```python
from build123d import *

# Parameters (mm, degrees)
BOSS_EXTRUDE3_DEPTH = 50
SKETCH7_R           = 30
BOSS_EXTRUDE4_DEPTH = 100
BOSS_EXTRUDE7_DEPTH = 500
SKETCH9_R           = 25
CUT_EXTRUDE1_DEPTH  = 500
CUT_EXTRUDE2_START  = -500
CUT_EXTRUDE2_DEPTH  = 500
FILLET1_R           = 10
SKETCH12_W          = 100
SKETCH12_H          = 20
BOSS_EXTRUDE8_DEPTH = 40
CUT_EXTRUDE3_DEPTH  = 40
SKETCH14_R          = 10
CUT_EXTRUDE4_DEPTH  = 40


with BuildPart() as part:
    # Sketch3 → Boss-Extrude3 (new body)
    with BuildSketch(Plane(origin=(0, 0, 0), x_dir=(0, 0, -1), z_dir=(1, 0, 0))):
        with BuildLine():
            Line((0, 30), (100, 30))
            ThreePointArc((100, 30), (130, 0), (100, -30))
            Line((100, -30), (0, -30))
            ThreePointArc((0, -30), (-30, 0), (0, 30))
        make_face()
    extrude(amount=BOSS_EXTRUDE3_DEPTH)

    # Sketch7 → Boss-Extrude4 (add)
    with BuildSketch(Plane(origin=(50, 0, 0), x_dir=(0, 0, -1), z_dir=(1, 0, 0))):
        with Locations(Location((100, 0, 0), (0, 0, 90))):
            Circle(SKETCH7_R)
    extrude(amount=BOSS_EXTRUDE4_DEPTH)

    # Sketch8 → Boss-Extrude7 (add)
    with BuildSketch(Plane(origin=(50, 0, 0), x_dir=(0, 0, -1), z_dir=(1, 0, 0))):
        with BuildLine():
            Line((0, 30), (20, 30))
            ThreePointArc((20, 30), (50, 0), (20, -30))
            Line((20, -30), (0, -30))
            ThreePointArc((0, -30), (-30, 0), (0, 30))
        make_face()
    extrude(amount=BOSS_EXTRUDE7_DEPTH)

    # Sketch9 → Cut-Extrude1 (cut)
    with BuildSketch(Plane(origin=(550, 0, 0), x_dir=(0, 0, -1), z_dir=(1, 0, 0))):
        with Locations((20, 0)):
            Circle(SKETCH9_R)
    extrude(amount=-CUT_EXTRUDE1_DEPTH, mode=Mode.SUBTRACT)

    # Sketch10 → Cut-Extrude2 (cut)
    with BuildSketch(Plane(origin=(550, 0, 0), x_dir=(0, 0, -1), z_dir=(1, 0, 0)).offset(CUT_EXTRUDE2_START)):
        with BuildLine():
            ThreePointArc((0, 30), (-15.932656638, 25.419489618), (-27, 13.076696831))
            Line((-27, 13.076696831), (12.529758535, 30))
            Line((12.529758535, 30), (0, 30))
        make_face()
        with BuildLine():
            Line((12.529758535, -30), (-27, -13.076696831))
            ThreePointArc((-27, -13.076696831), (-15.932656638, -25.419489618), (0, -30))
            Line((0, -30), (12.529758535, -30))
        make_face()
        with BuildLine():
            Line((-27, 0), (-27, 13.076696831))
            ThreePointArc((-27, 13.076696831), (-29.240383034, 6.708203932), (-30, 0))
            Line((-30, 0), (-27, 0))
        make_face()
        with BuildLine():
            Line((-27, -13.076696831), (-27, 0))
            Line((-27, 0), (-30, 0))
            ThreePointArc((-30, 0), (-29.240383034, -6.708203932), (-27, -13.076696831))
        make_face()
        with BuildLine():
            Line((-27, 0), (-27, 13.076696831))
            ThreePointArc((-27, 13.076696831), (-29.240383034, 6.708203932), (-30, 0))
            Line((-30, 0), (-27, 0))
        make_face()
        with BuildLine():
            Line((-27, -13.076696831), (-27, 0))
            Line((-27, 0), (-30, 0))
            ThreePointArc((-30, 0), (-29.240383034, -6.708203932), (-27, -13.076696831))
        make_face()
    extrude(amount=CUT_EXTRUDE2_DEPTH, mode=Mode.SUBTRACT)

    # Fillet1
    fillet1_edges = [part.edges().sort_by_distance(p)[0] for p in [
        (150, -30, -100),
    ]]
    fillet(fillet1_edges, radius=FILLET1_R)

    # Sketch12 → Boss-Extrude8 (add)
    with BuildSketch(Plane.ZY):
        with Locations((-50, -20)):
            Rectangle(SKETCH12_W, SKETCH12_H)
    extrude(amount=BOSS_EXTRUDE8_DEPTH)

    # Sketch13 → Cut-Extrude3 (cut)
    with BuildSketch(Plane.XZ.offset(30)):
        Polygon((-40, -35), (-25, 0), (-40, 0), align=None)
        Polygon((-40, -65), (-25, -100), (-40, -100), align=None)
    extrude(amount=-CUT_EXTRUDE3_DEPTH, mode=Mode.SUBTRACT)

    # Sketch14 → Cut-Extrude4 (cut)
    with BuildSketch(Plane(origin=(0, -30, 0), x_dir=(-1, 0, 0), z_dir=(0, -1, 0))):
        with Locations(Location((20, 25, 0), (0, 0, 90))):
            Circle(SKETCH14_R)
        with Locations(Location((20, 75, 0), (0, 0, 90))):
            Circle(SKETCH14_R)
    extrude(amount=-CUT_EXTRUDE4_DEPTH, mode=Mode.SUBTRACT)


solid = part.part
```
Source: CAD feature listing. Evaluate the final solid. Frame: model axes, mm. A direction names the side the tool comes from. Give positions to 0.01 mm unless a question says otherwise; leave off trailing zeros. Order: outer loops, then holes, each group sorted by start corner. A loop starts at its lowest first (then second) coordinate and runs counter-clockwise, first axis right, second up. Notation, with made-up numbers: (52.25, -18) -> (89.25, -18) arc R24 ccw to (89.25, -4) -> close; hole circle Ø5 at (49, -13.75). An arc over 180 degrees is marked (long way). Use a Markdown table: item, result.
Q1. Section A-A (x = -20). Return the cut outline in (y, z).
A:
| item | result |
|---|---|
| outline | (-30, -100) -> (-10, -100) -> (-10, -85) -> (-30, -85) -> close; (-30, -65) -> (-10, -65) -> (-10, -35) -> (-30, -35) -> close; (-30, -15) -> (-10, -15) -> (-10, 0) -> (-30, 0) -> close |
Q2. Section C-C (y = 0). Return the cut outline in (x, z).
A:
| item | result |
|---|---|
| outline | (0, -130) -> (140, -130) arc R10 ccw to (150, -120) -> (150, -80) arc R10 ccw to (140, -70) -> (50, -70) -> (50, -50) -> (550, -50) -> (550, -45) -> (50, -45) -> (50, 5) -> (550, 5) -> (550, 27) -> (50, 27) -> (50, 30) -> (0, 30) -> close |
Q3. Pull-direction query (X, two-part tool) for faces 1 (the face through (-17, -20.14, -34.54)), 2 (the face through (296.5, 21.42, 7.51)), 3 (the face through (-32.605, -20.14, -17.745)), 4 (the face through (50, 23, 9)); classes: +X half, -X half, draft (parallel to the pull), parting line (faces both ways), or undercut.
A:
| item | result |
|---|---|
| face 1 | undercut |
| face 2 | draft |
| face 3 | -X half |
| face 4 | +X half |
Q4. Section B-B (x = 207). Return the cut outline in (y, z).
A:
| item | result |
|---|---|
| outline | (-30, -20) arc R30 ccw to (30, -20) -> (30, -12.53) -> (13.08, 27) -> (-13.08, 27) -> (-30, -12.53) -> close; hole circle Ø50 at (0, -20) |
Q5. Material intervals for line 1 (Y direction, x = 326.5, z = -20); line 2 (Z direction, x = 106.5, y = -9.5); line 3 (X direction, y = -4.5, z = -113), sorted ascending. Write a range as [from, to].
A:
| item | result |
|---|---|
| line 1 | [-30, -25], [25, 30] |
| line 2 | [-128.46, -71.54], [-48.46, -43.12], [3.12, 27] |
| line 3 | [0, 150] |
Q6. First-contact query: P1, Ø5, axis at x = 384, z = 4.5, coming from the -Y side; P2, Ø20, axis at y = 1.5, z = -106.5, coming from the +X side; P3, Ø10, axis at x = 435, z = -47, coming from the -Y side; P4, Ø18, axis at x = -20, z = -25, coming from the -Y side. Flat tips, straight axial feed; report the tip coordinate or a pass-through.
A:
| item | result |
|---|---|
| P1 | y = -23.78 |
| P2 | x = 150 |
| P3 | y = -20.4 |
| P4 | through |
Q7. Access query for faces 5 (the face through (296, 0, 27)), 6 (the face through (296.5, -21.657, 6.958)), 7 (the face through (296.5, 0.66, -49.993)). Directions: +Z, -Z, +X, -X, +Y, -Y. A direction counts if a zero-diameter tool reaches every point of the face in a straight line with its end or side. Return the directions, or none.
A:
| item | result |
|---|---|
| face 5 | +Z, +X, +Y, -Y |
| face 6 | +Z, +X, -Y |
| face 7 | +X |
Q8. Section D-D (z = -25). Return the cut outline in (x, y).
A:
| item | result |
|---|---|
| outline | (-35.71, -30) -> (-30, -30) -> (-30, -10) -> (-35.71, -10) -> close; (-10, -30) -> (50, -30) -> (50, -29.58) -> (550, -29.58) -> (550, -24.49) -> (50, -24.49) -> (50, 24.49) -> (550, 24.49) -> (550, 29.58) -> (50, 29.58) -> (50, 30) -> (0, 30) -> (0, -10) -> (-10, -10) -> close |
